from build123d import *

# Parameters (mm, degrees)
BOSS_EXTRUDE1_DEPTH = 2.5
FILLET1_R           = 16
FILLET2_R           = 6.3
BOSS_EXTRUDE2_DEPTH = 14.5
FILLET3_R           = 1
SKETCH5_W           = 5.5
SKETCH5_H           = 5.5
CUT_EXTRUDE1_DEPTH  = 31.959805
SKETCH6_R           = 1.55
CUT_EXTRUDE2_DEPTH  = 2.5
SKETCH7_R           = 1.55
CUT_EXTRUDE3_DEPTH  = 2.5


with BuildPart() as part:
    # Sketch1 → Boss-Extrude1 (new body)
    with BuildSketch(Plane(origin=(0, 0, 0), x_dir=(1, 0, 0), z_dir=(0, 1, 0))):
        Polygon((0, 12.577166077), (-40.072620247, 0), (0, -12.577166077), (40.072620247, 0), align=None)
    extrude(amount=BOSS_EXTRUDE1_DEPTH)

    # Fillet1
    fillet1_edges = [part.edges().sort_by_distance(p)[0] for p in [
        (0, 1.25, 12.577166077),
        (0, 1.25, -12.577166077),
    ]]
    fillet(fillet1_edges, radius=FILLET1_R)

    # Fillet2
    fillet2_edges = [part.edges().sort_by_distance(p)[0] for p in [
        (40.072620247, 1.25, 0),
        (-40.072620247, 1.25, 0),
    ]]
    fillet(fillet2_edges, radius=FILLET2_R)

    # Sketch2 → Boss-Extrude2 (add)
    with BuildSketch(Plane(origin=(0, 2.5, 0), x_dir=(1, 0, 0), z_dir=(0, 1, 0))):
        Polygon((2, 2), (11.5, 2), (11.5, -2), (2, -2), (2, -11.5), (-2, -11.5), (-2, -2), (-11.5, -2), (-11.5, 2), (-2, 2), (-2, 11.5), (2, 11.5), align=None)
    extrude(amount=BOSS_EXTRUDE2_DEPTH)

    # Sketch3 → Cut-Revolve1 (revolve, cut)
    with BuildSketch(Plane.XY):
        with BuildLine():
            ThreePointArc((0, 4.5), (7.9, 12.4), (0, 20.3))
            Line((0, 20.3), (0, 4.5))
        make_face()
    revolve(axis=Axis((0, 20.3, 0), (0, -1, 0)), mode=Mode.SUBTRACT)

    # Fillet3
    fillet3_edges = [part.edges().sort_by_distance(p)[0] for p in [
        (-11.5, 17, 0),
        (0, 17, 11.5),
        (11.5, 17, 0),
        (0, 17, -11.5),
    ]]
    fillet(fillet3_edges, radius=FILLET3_R)

    # Sketch5 → Cut-Extrude1 (cut)
    with BuildSketch(Plane(origin=(0, 2.5, 0), x_dir=(1, 0, 0), z_dir=(0, 1, 0))):
        Rectangle(SKETCH5_W, SKETCH5_H)
    extrude(amount=CUT_EXTRUDE1_DEPTH, mode=Mode.SUBTRACT)

    # Sketch6 → Cut-Extrude2 (cut)
    with BuildSketch(Plane(origin=(0, 2.5, 0), x_dir=(1, 0, 0), z_dir=(0, 1, 0))):
        Circle(SKETCH6_R)
    extrude(amount=-CUT_EXTRUDE2_DEPTH, mode=Mode.SUBTRACT)

    # Sketch7 → Cut-Extrude3 (cut)
    with BuildSketch(Plane(origin=(0, 2.5, 0), x_dir=(1, 0, 0), z_dir=(0, 1, 0))):
        with Locations((20.32, 0)):
            Circle(SKETCH7_R)
        with Locations((-20.32, 0)):
            Circle(SKETCH7_R)
    extrude(amount=-CUT_EXTRUDE3_DEPTH, mode=Mode.SUBTRACT)


solid = part.part
Can you work these out from the model? Positions are in its coordinate system, mm. A direction names the side the tool comes from. Give positions to 0.01 mm unless a question says otherwise; leave off trailing zeros. Write each loop counter-clockwise with the first axis right and the second up, starting at its lowest first coordinate (ties: lowest second). Pieces come first, ordered by that corner, then holes. Notation, with made-up numbers: (42.5, 1.25) -> (78.5, 1.25) arc R20 cw to (78.5, 8.25) -> close; hole circle Ø8 at (12.5, -29). An arc over 180 degrees is marked (long way). Answer as a JSON object with one key per item and string values. Group by question number.
Item 1: We'd pull the mould along X, two halves only. Please class faces 1 (the face through (-0.068, 1.268, 11.807)), 2 (the face through (0, 0, -3)), 3 (the face through (-2, 8, -8)), 4 (the face through (-2.75, 4, 0)): +X half, -X half, draft (parallel to the pull), parting line (faces both ways), or undercut.
Item 2: Suppose I cut it at C-C (y = 12.75). Please give me the cut outline in (x, z), plus the area to 3 significant figures.
Item 3: I'm going to push flat-ended pins straight in: P1, Ø4, axis at x = 0, z = -4, coming from the +Y side; P2, Ø7, axis at x = -8, y = 7.5, coming from the -Z side; P3, Ø4, axis at y = 9.5, z = -7, coming from the +X side. Where does each tip first touch, or does it pass through?
Item 4: Please list where these lines run through material, in increasing order: line 1 (X direction, y = 0.9, z = 0); line 2 (Z direction, x = 0, y = 1.8); line 3 (Y direction, x = 21, z = -5.75). Write a range as [from, to].
Item 5: Suppose I cut it at A-A (z = -7.25). Please give me the cut outline in (x, y), plus the area to 3 significant figures.
Item 6: Suppose I cut it at B-B (x = 0). Please give me the cut outline in (y, z).
Item 7: Suppose I cut it at D-D (z = 0). Please give me the cut outline in (x, y).
Item 8: For faces 5 (the face through (11.5, 9, 0)), 6 (the face through (8, 8, -2)), 7 (the face through (2.75, 4, 0)), which set-ups out of +Z, -Z, +X, -X, +Y, -Y let a thin tool reach every point of the face, with its end or its side?
Findings:
{
 "1": {"face 1": "parting line", "face 2": "draft", "face 3": "-X half", "face 4": "undercut"},
 "2": {"outline": "(-11.5, -2) -> (-7.63, -2) arc R7.89 cw to (-7.63, 2) -> (-11.5, 2) -> close; (-2, -11.5) -> (2, -11.5) -> (2, -7.63) arc R7.89 cw to (-2, -7.63) -> close; (-2, 7.63) arc R7.89 cw to (2, 7.63) -> (2, 11.5) -> (-2, 11.5) -> close; (7.63, -2) -> (11.5, -2) -> (11.5, 2) -> (7.63, 2) arc R7.89 cw to start", "area": "59.1 mm²"},
 "3": {"P1": "stops at y = 7.26", "P2": "stops at z = -2", "P3": "stops at x = 2"},
 "4": {"line 1": "x = [-25.33, -21.87], [-18.77, -1.55], [1.55, 18.77], [21.87, 25.33]", "line 2": "z = [-11.81, -1.55], [1.55, 11.81]", "line 3": "y = [0, 2.5]"},
 "5": {"outline": "(-16.97, 0) -> (16.97, 0) -> (16.97, 2.5) -> (2, 2.5) -> (2, 9.98) arc R3.14 cw to (-2, 9.98) -> (-2, 2.5) -> (-16.97, 2.5) -> close; (-2, 14.82) arc R3.14 cw to (2, 14.82) -> (2, 17) -> (-2, 17) -> close", "area": "120 mm²"},
 "6": {"outline": "(0, -11.81) -> (2.5, -11.81) -> (2.5, -11.5) -> (16, -11.5) arc R1 ccw to (17, -10.5) -> (17, -6.42) arc R7.9 cw to (4.99, -2.75) -> (2.5, -2.75) -> (2.5, -1.55) -> (0, -1.55) -> close; (0, 1.55) -> (2.5, 1.55) -> (2.5, 2.75) -> (4.99, 2.75) arc R7.9 cw to (17, 6.42) -> (17, 10.5) arc R1 ccw to (16, 11.5) -> (2.5, 11.5) -> (2.5, 11.81) -> (0, 11.81) -> close"},
 "7": {"outline": "(-25.33, 0) -> (-21.87, 0) -> (-21.87, 2.5) -> (-25.33, 2.5) -> close; (-18.77, 0) -> (-1.55, 0) -> (-1.55, 2.5) -> (-2.75, 2.5) -> (-2.75, 4.99) arc R7.9 cw to (-6.42, 17) -> (-10.5, 17) arc R1 ccw to (-11.5, 16) -> (-11.5, 2.5) -> (-18.77, 2.5) -> close; (1.55, 0) -> (18.77, 0) -> (18.77, 2.5) -> (11.5, 2.5) -> (11.5, 16) arc R1 ccw to (10.5, 17) -> (6.42, 17) arc R7.9 cw to (2.75, 4.99) -> (2.75, 2.5) -> (1.55, 2.5) -> close; (21.87, 0) -> (25.33, 0) -> (25.33, 2.5) -> (21.87, 2.5) -> close"},
 "8": {"face 5": "+Z, -Z, +X, +Y", "face 6": "-Z, +X, -X, +Y", "face 7": "+Z, -Z, +Y"}
}
